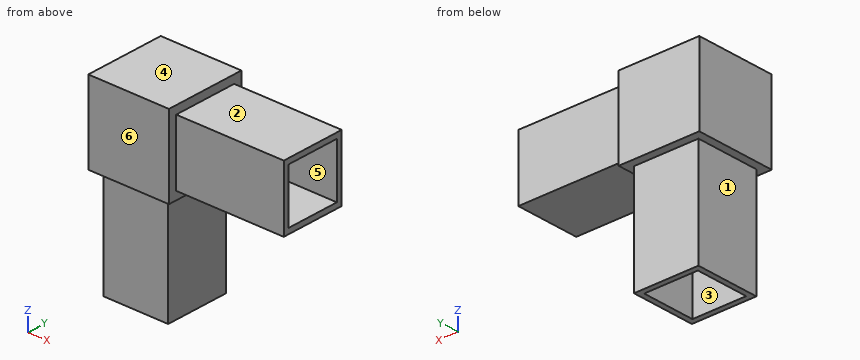
from build123d import *

# Parameters (mm, degrees)
CROQUIS1_W     = 30
CROQUIS1_H     = 40
CROQUIS1_H_2   = 30
CROQUIS1_W_2   = 40
EXTRUIR1_DEPTH = 30
CROQUIS2_W     = 30
CROQUIS2_H     = 30
CROQUIS2_W_2   = 24
CROQUIS2_H_2   = 24
EXTRUIR2_DEPTH = 40
CROQUIS3_W     = 30
CROQUIS3_H     = 30
CROQUIS3_W_2   = 24
CROQUIS3_H_2   = 24
EXTRUIR3_DEPTH = 40
VACIADO1_T     = -2


with BuildPart() as part:
    # Croquis1 → Extruir1 (new body)
    with BuildSketch(Plane(origin=(0, 0, 0), x_dir=(1, 0, 0), z_dir=(0, 1, 0))):
        with Locations((0, 35)):
            Rectangle(CROQUIS1_W, CROQUIS1_H)
        Rectangle(CROQUIS1_W, CROQUIS1_H_2)
        with Locations((35, 0)):
            Rectangle(CROQUIS1_W_2, CROQUIS1_H_2)
    extrude(amount=EXTRUIR1_DEPTH)

    # Croquis2 → Extruir2 (cut)
    with BuildSketch(Plane(origin=(55, 0, 0), x_dir=(0, 0, -1), z_dir=(1, 0, 0))):
        with Locations((0, 15)):
            Rectangle(CROQUIS2_W, CROQUIS2_H)
        with Locations((0, 15)):
            Rectangle(CROQUIS2_W_2, CROQUIS2_H_2, mode=Mode.SUBTRACT)
    extrude(amount=-EXTRUIR2_DEPTH, mode=Mode.SUBTRACT)

    # Croquis3 → Extruir3 (cut)
    with BuildSketch(Plane(origin=(0, 0, -55), x_dir=(-1, 0, 0), z_dir=(0, 0, -1))):
        with Locations((0, 15)):
            Rectangle(CROQUIS3_W, CROQUIS3_H)
        with Locations((0, 15)):
            Rectangle(CROQUIS3_W_2, CROQUIS3_H_2, mode=Mode.SUBTRACT)
    extrude(amount=-EXTRUIR3_DEPTH, mode=Mode.SUBTRACT)

    # Vaciado1
    vaciado1_openings = [part.faces().sort_by_distance(p)[0] for p in [
        (55, 15, 0),
        (0, 15, -55),
    ]]
    offset(amount=VACIADO1_T, openings=vaciado1_openings, kind=Kind.INTERSECTION)


solid = part.part
Part model, mm, in its own coordinate system. Face numbers are marked on the shaded views. A direction names the side the tool comes from. Give positions to 0.01 mm unless a question says otherwise; leave off trailing zeros. Order: outer loops, then holes, each group sorted by start corner. A loop starts at its lowest first (then second) coordinate and runs counter-clockwise, first axis right, second up. Notation, with made-up numbers: (82, 8) - (124, 8) arc R19 ccw to (124, 37) - close; hole circle Ø3 at (-0.75, 41). An arc over 180 degrees is marked (long way). Use a Markdown table: item, result.
1) Saw through at B-B on y = 24. List the corners of the cut face in (x, z), plus the area to 3 significant figures.
Checked values:
| item | result |
|---|---|
| outline | (-15, -15) - (-12, -15) - (-12, -55) - (-10, -55) - (-10, -13) - (-13, -13) - (-13, 13) - (13, 13) - (13, 10) - (55, 10) - (55, 12) - (15, 12) - (15, 15) - (-15, 15) - close; (10, -55) - (12, -55) - (12, -15) - (15, -15) - (15, -12) - (55, -12) - (55, -10) - (13, -10) - (13, -13) - (10, -13) - close |
| area | 464 mm² |
2) Saw through at D-D on z = -7.5. List the corners of the cut face in (x, y), plus the area to 3 significant figures.
Checked values:
| item | result |
|---|---|
| outline | (-15, 0) - (15, 0) - (15, 3) - (55, 3) - (55, 5) - (13, 5) - (13, 2) - (-13, 2) - (-13, 28) - (13, 28) - (13, 25) - (55, 25) - (55, 27) - (15, 27) - (15, 30) - (-15, 30) - close |
| area | 344 mm² |
3) Probe L1, parallel to Y at x = 16, z = -6.5; L2, parallel to Y at x = 12.5, z = 8.5; L3, parallel to X at y = 21.75, z = -25.5. List the from-to ranges inside material, lowest first. Write a range as from..to.
Checked values:
| item | result |
|---|---|
| L1 | 3..5, 25..27 |
| L2 | 0..2, 28..30 |
| L3 | -12..-10, 10..12 |
4) Two-plate mould, pull along Y, no slides. Class the marked faces 4, 5 and 6: +Y half, -Y half, draft (parallel to the pull), parting line (faces both ways), or undercut.
Checked values:
| item | result |
|---|---|
| face 4 | draft |
| face 5 | undercut |
| face 6 | -Y half |
5) Saw through at C-C on z = -19.5. List the corners of the cut face in (x, y), plus the area to 3 significant figures.
Checked values:
| item | result |
|---|---|
| outline | (-12, 3) - (12, 3) - (12, 27) - (-12, 27) - close; hole (-10, 5) - (10, 5) - (10, 25) - (-10, 25) - close |
| area | 176 mm² |
6) Flat gauge pins, fed straight in: P1, Ø19, axis at x = -1.5, z = -26.5, coming from the -Y side; P2, Ø2, axis at y = 11, z = -39.5, coming from the +X side; P3, Ø7, axis at x = 26.5, z = -1, coming from the +Y side. Where does each tip first touch, or does it go through?
Checked values:
| item | result |
|---|---|
| P1 | y = 3 |
| P2 | x = 12 |
| P3 | y = 27 |
7) Saw through at A-A on x = 38.5. List the corners of the cut face in (y, z).
Checked values:
| item | result |
|---|---|
| outline | (3, -12) - (27, -12) - (27, 12) - (3, 12) - close; hole (5, -10) - (25, -10) - (25, 10) - (5, 10) - close |
8) 3-axis set-ups, long thin cutter, end or side, ignore diameter. For the marked faces 1, 2 and 3: which of +Z, -Z, +X, -X, +Y, -Y reach the whole face in a straight line?
Checked values:
| item | result |
|---|---|
| face 1 | -Z, -X, +Y, -Y |
| face 2 | +Z, +X, +Y, -Y |
| face 3 | -Z |
